Build history of the part. All positions in model axes, mm. Face numbers are marked on the shaded views. Coordinates: 2 decimals unless noted, no trailing zeros. Order: outer loops, then holes, each group sorted by start corner. A loop starts at its lowest first (then second) coordinate and runs counter-clockwise, first axis right, second up. Notation, with made-up numbers: M -40,-38.75 L -21,-38.75 A28 cw -21,-19.75 Z; hole C 88,87.5 d7. An arc over 180 degrees is marked long. Use a Markdown table: item, result. Add a question column.
from build123d import *

# Parameters (mm, degrees)
SKETCH1_R                = 10
BOSS_EXTRUDE1_DEPTH      = 15
SKETCH2_R                = 9
SKETCH2_R_2              = 4
CUT_EXTRUDE1_DEPTH       = 1
M3_CLEARANCE_HOLE1_D     = 3.2
M3_CLEARANCE_HOLE1_DEPTH = 5
M3_CLEARANCE_HOLE1_TIP   = 0.96137699


with BuildPart() as part:
    # Sketch1 → Boss-Extrude1 (new body)
    with BuildSketch(Plane(origin=(0, 0, 0), x_dir=(1, 0, 0), z_dir=(0, 1, 0))):
        with Locations(Location((0, 0, 0), (0, 0, 270))):
            Circle(SKETCH1_R)
    extrude(amount=BOSS_EXTRUDE1_DEPTH)

    # Sketch2 → Cut-Extrude1 (cut)
    with BuildSketch(Plane(origin=(0, 15, 0), x_dir=(1, 0, 0), z_dir=(0, 1, 0))):
        with Locations(Location((0, 0, 0), (0, 0, 270))):
            Circle(SKETCH2_R)
        with Locations(Location((0, 0, 0), (0, 0, 270))):
            Circle(SKETCH2_R_2, mode=Mode.SUBTRACT)
    extrude(amount=-CUT_EXTRUDE1_DEPTH, mode=Mode.SUBTRACT)

    # M3 Clearance Hole1
    with Locations(Plane(origin=(0, 0, 0), x_dir=(-1, 0, 0), z_dir=(0, -1, 0))):
        with Locations((0, 0)):
            Hole(M3_CLEARANCE_HOLE1_D / 2, depth=M3_CLEARANCE_HOLE1_DEPTH)
            with Locations((0, 0, -(M3_CLEARANCE_HOLE1_DEPTH + M3_CLEARANCE_HOLE1_TIP / 2))):  # 118° drill point
                Cone(0, M3_CLEARANCE_HOLE1_D / 2, M3_CLEARANCE_HOLE1_TIP, mode=Mode.SUBTRACT)


solid = part.part
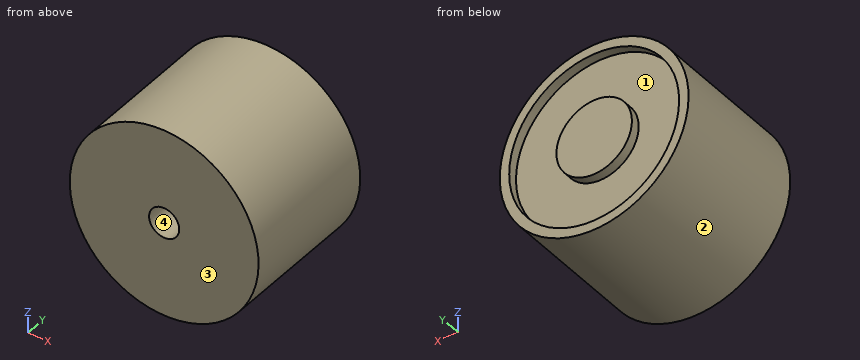
(1) Slice it at A-A on y = 1.25. Give the cut face in (x, z).
(2) Slice it at B-B on x = -6. Give the cut face in (y, z), and give its area (3 significant figures).
(3) Mould opens along X. For the marked faces 1, 2, 3 and 4 say: released by +X, released by -X, zero draft, split by the parting line, or undercut.
(4) Drop flat-ended pins along their axis: P1, Ø6, axis at y = 13, z = -3.5, coming from the -X side; P2, Ø1.5, axis at x = 6, y = 12, coming from the -Z side; P3, Ø1, axis at x = -4, y = 12, coming from the -Z side. Give the stop position or say it passes through.
(5) Drill centre lines: line 1 along X through (y, z) = (14.45, 0); line 2 along Y through (x, z) = (1.25, 7.25); line 3 along X through (y, z) = (14.25, 5.75). Where is each one in solid material? Low to high. Write a range as from..to.
(6) Slice it at D-D on y = 12.25. Give the cut face in (x, z), and give its area (3 significant figures).
(7) Slice it at C-C on z = 5.5. Give the cut face in (x, y), and give its area (3 significant figures).
Solutions:
| question | item | result |
|---|---|---|
| 1 | outline | C 0,0 d20; hole C 0,0 d3.2 |
| 2 | outline | M 0,-8 L 15,-8 L 15,-6.71 L 14,-6.71 L 14,6.71 L 15,6.71 L 15,8 L 0,8 Z |
| 2 | area | 227 mm² |
| 3 | face 1 | undercut |
| 3 | face 2 | split by the parting line |
| 3 | face 3 | zero draft |
| 3 | face 4 | undercut |
| 4 | P1 | x = -9.99 |
| 4 | P2 | z = -8.51 |
| 4 | P3 | z = -9.37 |
| 5 | line 1 | -10..-9, -4..4, 9..10 |
| 5 | line 2 | 0..14 |
| 5 | line 3 | -8.18..-6.92, 6.92..8.18 |
| 6 | outline | C 0,0 d20 |
| 6 | area | 314 mm² |
| 7 | outline | M -8.35,0 L 8.35,0 L 8.35,15 L 7.12,15 L 7.12,14 L -7.12,14 L -7.12,15 L -8.35,15 Z |
| 7 | area | 236 mm² |
